For this review, take the finished solid that the model builds, in its own axes (mm). Face numbers are marked on the shaded views. A direction names the side the tool comes from. Round coordinates to 2 decimals unless told otherwise and drop trailing zeros. Order: outer loops, then holes, each group sorted by start corner. A loop starts at its lowest first (then second) coordinate and runs counter-clockwise, first axis right, second up. Notation, with made-up numbers: (11.5, 9.5) -> (47.5, 9.5) arc R5 cw to (47.5, 14.5) -> close; hole circle Ø3 at (14, 48). An arc over 180 degrees is marked (long way). Answer in a Markdown table with one row per item.
```python
from build123d import *

# Parameters (mm, degrees)
BASPROSKE_W        = 10.5
BASPROSKE_H        = 10.5
TOOTHCUT_DEPTH     = 19.186533479
TEETHCUTS_COUNT    = 12
TEETHCUTS_ANGLE    = 330
BORSKE_R           = 0.5
BORE_DEPTH         = 50.0000508
SKETCH1_W          = 3.2
SKETCH1_H          = 3.2
CUT_EXTRUDE1_DEPTH = 30


with BuildPart() as part:
    # BasProSke → Base-Revolve (revolve)
    with BuildSketch(Plane(origin=(0, 0, 0), x_dir=(1, 0, 0), z_dir=(0, 1, 0)), mode=Mode.PRIVATE) as base_revolve_sk:
        with Locations((5.25, 5.25)):
            Rectangle(BASPROSKE_W, BASPROSKE_H)
    revolve(base_revolve_sk.sketch.rotate(Axis((-10, 0, 0), (1, 0, 0)), 180), axis=Axis((-10, 0, 0), (1, 0, 0)))

    # TooCutSke → ToothCut (cut, through all)
    with BuildSketch(Plane(origin=(0, 0, 0), x_dir=(0, 0, -1), z_dir=(1, 0, 0))):
        with BuildLine():
            ThreePointArc((0.837751456, 7.074570552), (0, 7.124), (-0.837751456, 7.074570552))
            ThreePointArc((-0.837751456, 7.074570552), (-1.245380016, 8.868946541), (-2.486473743, 10.227487154))
            ThreePointArc((-2.486473743, 10.227487154), (0, 10.5254), (2.486473743, 10.227487154))
            ThreePointArc((2.486473743, 10.227487154), (1.245380016, 8.868946541), (0.837751456, 7.074570552))
        make_face()
    toothcut = extrude(amount=TOOTHCUT_DEPTH, mode=Mode.SUBTRACT)

    # TeethCuts: ToothCut ×12 about axis
    teethcuts_axis = Axis((-10, 0, 0), (1, 0, 0))
    for i in range(1, TEETHCUTS_COUNT):
        add(toothcut.rotate(teethcuts_axis, i * TEETHCUTS_ANGLE / (TEETHCUTS_COUNT - 1)), mode=Mode.SUBTRACT)

    # BorSke → Bore (cut, symmetric)
    with BuildSketch(Plane(origin=(0, 0, 0), x_dir=(0, 0, -1), z_dir=(1, 0, 0))):
        with Locations(Location((0, 0, 0), (0, 0, 180))):
            Circle(BORSKE_R)
    extrude(amount=BORE_DEPTH, both=True, mode=Mode.SUBTRACT)

    # Sketch1 → Cut-Extrude1 (cut)
    with BuildSketch(Plane(origin=(10.5, 0, 0), x_dir=(0, 0, -1), z_dir=(1, 0, 0))):
        Rectangle(SKETCH1_W, SKETCH1_H)
    extrude(amount=-CUT_EXTRUDE1_DEPTH, mode=Mode.SUBTRACT)


solid = part.part
```
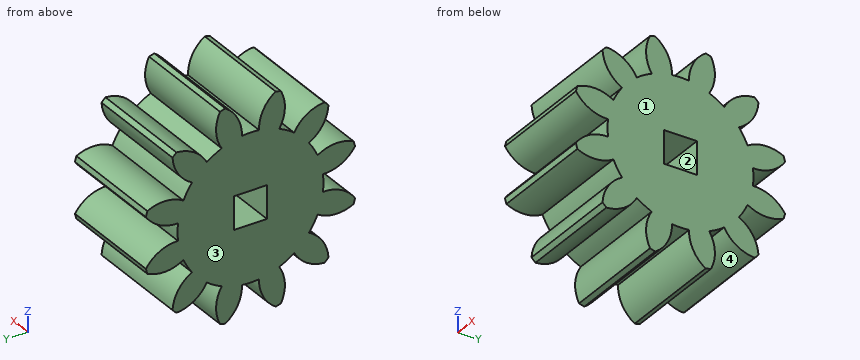
Q1. Take a section at C-C, the plane z = 5.25. Write out the cut boundary in (x, y), then the cut area to 3 significant figures.
Answer key:
| item | result |
|---|---|
| outline | (0, -6.87) -> (10.5, -6.87) -> (10.5, 6.87) -> (0, 6.87) -> close |
| area | 144 mm^2 |
Q2. Take a section at A-A, the plane y = -8.25. Write out the cut boundary in (x, z).
Answer key:
| item | result |
|---|---|
| outline | (0, -3.35) -> (10.5, -3.35) -> (10.5, -0.99) -> (0, -0.99) -> close; (0, 0.99) -> (10.5, 0.99) -> (10.5, 3.35) -> (0, 3.35) -> close |
Q3. Take a section at D-D, the plane z = 2. Write out the cut boundary in (x, y), then the cut area to 3 significant figures.
Answer key:
| item | result |
|---|---|
| outline | (0, -9.85) -> (10.5, -9.85) -> (10.5, 9.85) -> (0, 9.85) -> close |
| area | 207 mm^2 |
Q4. Tool access review of the marked faces 1 and 2: name each direction out of +Z, -Z, +X, -X, +Y, -Y from which nothing blocks a thin tool from reaching the whole face with its end or side.
Answer key:
| item | result |
|---|---|
| face 1 | +Z, -Z, +X, +Y, -Y |
| face 2 | +X, -X |
Q5. Clearance check with flat-ended pins moving along their axes: pin 1 Ø1 at (x, z) = (2.5, 5) entering from +Y; pin 2 Ø3 at (x, y) = (7.5, 1.5) entering from -Z; pin 3 Ø3.5 at (x, y) = (3.5, -0.5) entering from -Z. State where each tip first meets the part, or that it passes through.
Answer key:
| item | result |
|---|---|
| pin 1 | stops at y = 7.05 |
| pin 2 | stops at z = -10.21 |
| pin 3 | stops at z = -10.06 |
Q6. To check wall thickness, follow probe 1 along Z at (x, y) = (2, 6); probe 2 along Y at (x, z) = (2.75, 0); probe 3 along Z at (x, y) = (6.5, 6.75). State the ranges of each line that lie inside material, in increasing order.
Answer key:
| item | result |
|---|---|
| probe 1 | z = -7.32 to -4.44, -3.84 to 3.84, 4.44 to 7.32 |
| probe 2 | y = -7.12 to -1.6, 1.6 to 7.12 |
| probe 3 | z = -7.55 to -5.1, -2.93 to 2.93, 5.1 to 7.55 |
Q7. The part is to be moulded in two halves that separate along Y. For the marked faces 3 and 4, say which applies: +Y half, -Y half, draft (parallel to the pull), parting line (faces both ways), or undercut.
Answer key:
| item | result |
|---|---|
| face 3 | draft |
| face 4 | undercut |
Q8. Take a section at B-B, the plane z = -1.25. Write out the cut boundary in (x, y).
Answer key:
| item | result |
|---|---|
| outline | (0, -8.88) -> (10.5, -8.88) -> (10.5, -1.6) -> (0, -1.6) -> close; (0, 1.6) -> (10.5, 1.6) -> (10.5, 8.88) -> (0, 8.88) -> close |
